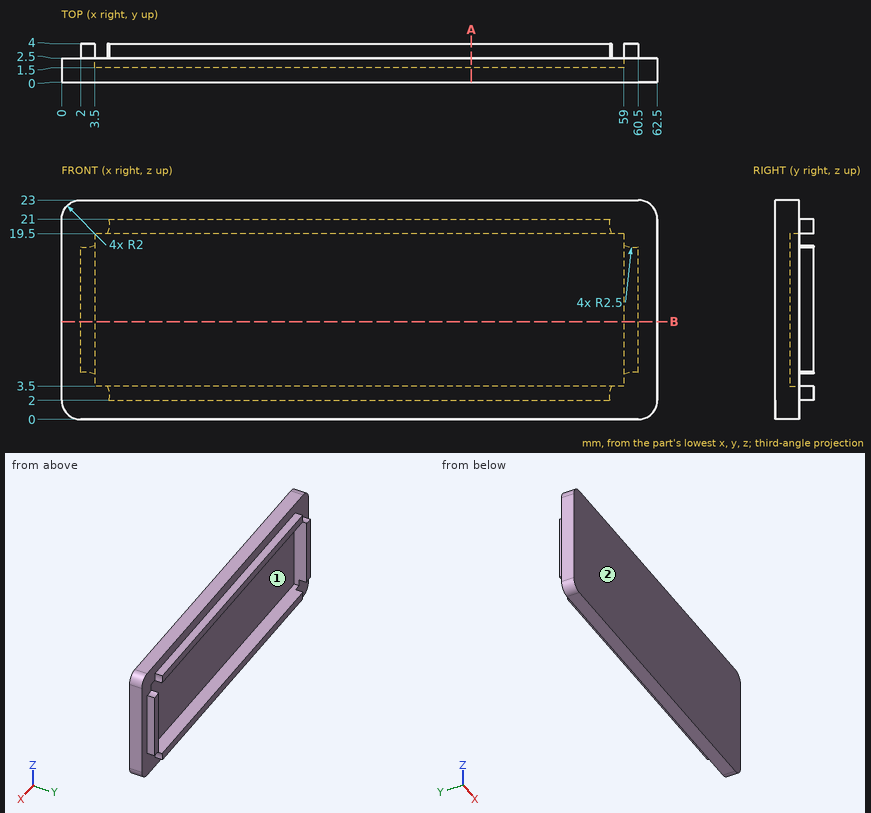
Study the drawing (mm; zero at the part's minimum x, y, z) and answer. Round coordinates to 2 decimals unless told otherwise and drop trailing zeros. Write each loop counter-clockwise with the first axis right and the second up, starting at its lowest first coordinate (ties: lowest second). Pieces come first, ordered by that corner, then holes.
1) The mould has two halves that part along X. Classify the marked faces 1 and 2: pulls with the +X half, pulls with the -X half, needs draft (parallel to the pull), parting line crosses it, or undercut.
2) Straight lines are drawn through the part: line 1 (Z direction, x = 8.5, y = 2.95); line 2 (X direction, y = 3.75, z = 11.75); line 3 (X direction, y = 2.35, z = 12.75). For each, find the intervals that lie inside material, in ascending order.
3) A cutting plane is placed at B-B (z = 10.25). Give the vertices of the cut face in (x, y).
4) Given pin 1 Ø1.6 at (x, y) = (30, 3.5) entering from +Z; pin 2 Ø1.6 at (y, z) = (3.5, 8.5) entering from -X; pin 3 Ø3 at (x, z) = (43, 7.5) entering from +Y, each flat-ended and moving along its own axis, determine where each tip first touches the part or whether it passes through.
5) A cutting plane is placed at A-A (x = 43). Give the vertices of the cut face in (y, z).
Completed:
1. face 1: undercut
1. face 2: needs draft
2. line 1: z = 2 to 3.5, 19.5 to 21
2. line 2: x = 2 to 3.5, 59 to 60.5
2. line 3: x = 0 to 3.5, 59 to 62.5
3. outline: (0, 0) - (62.5, 0) - (62.5, 2.5) - (60.5, 2.5) - (60.5, 4) - (59, 4) - (59, 1.5) - (3.5, 1.5) - (3.5, 4) - (2, 4) - (2, 2.5) - (0, 2.5) - close
4. pin 1: stops at z = 21
4. pin 2: stops at x = 2
4. pin 3: stops at y = 1.5
5. outline: (0, 0) - (2.5, 0) - (2.5, 2) - (4, 2) - (4, 3.5) - (1.5, 3.5) - (1.5, 19.5) - (4, 19.5) - (4, 21) - (2.5, 21) - (2.5, 23) - (0, 23) - close
